Check sheet for the modelled part. Datum: model origin and axes. Units: mm. Give positions to 0.01 mm unless a question says otherwise; leave off trailing zeros. Order: outer loops, then holes, each group sorted by start corner. A loop starts at its lowest first (then second) coordinate and runs counter-clockwise, first axis right, second up. Notation, with made-up numbers: M 78.25,29 L 106.25,29 A7 ccw 106.25,36 Z; hole C -25,6.5 d2. An arc over 180 degrees is marked long. Return JSON: item names as keys, results as strings. Group by question number.
from build123d import *

# Parameters (mm, degrees)
BOSS_EXTRUDE1_DEPTH = 3
SKETCH2_W           = 249.6
SKETCH2_H           = 3
SKETCH2_W_2         = 14.577777778
SKETCH2_W_3         = 14.577777777
BOSS_EXTRUDE2_DEPTH = 3
BOSS_EXTRUDE5_DEPTH = 3
BOSS_EXTRUDE4_DEPTH = 3


with BuildPart() as part:
    # Sketch1 → Boss-Extrude1 (new body)
    with BuildSketch(Plane.XY):
        Polygon((-124.8, 111.588319146), (124.8, 111.588319146), (65, -111.588319146), (-65, -111.588319146), align=None)
    extrude(amount=BOSS_EXTRUDE1_DEPTH)

    # Sketch2 → Boss-Extrude2 (add, through all)
    with BuildSketch(Plane.XY.offset(3)):
        with Locations((0, 113.088319146)):
            Rectangle(SKETCH2_W, SKETCH2_H)
        with Locations((-57.711111111, -113.088319146)):
            Rectangle(SKETCH2_W_2, SKETCH2_H)
        with Locations((-28.855555556, -113.088319146)):
            Rectangle(SKETCH2_W_3, SKETCH2_H)
        with Locations((0, -113.088319146)):
            Rectangle(SKETCH2_W_2, SKETCH2_H)
        with Locations((28.855555556, -113.088319146)):
            Rectangle(SKETCH2_W_3, SKETCH2_H)
        with Locations((57.711111111, -113.088319146)):
            Rectangle(SKETCH2_W_2, SKETCH2_H)
    extrude(amount=-BOSS_EXTRUDE2_DEPTH)

    # Sketch4 → Boss-Extrude5 (add, through all)
    with BuildSketch(Plane.XY.offset(3)):
        Polygon((-124.8, 140.588319146), (-97.2, 140.588319146), (-97.2, 143.588319146), (-69.3, 143.588319146), (-69.3, 140.588319146), (-41.7, 140.588319146), (-41.7, 143.588319146), (-13.8, 143.588319146), (-13.8, 140.588319146), (13.8, 140.588319146), (13.8, 143.588319146), (41.7, 143.588319146), (41.7, 140.588319146), (69.3, 140.588319146), (69.3, 143.588319146), (97.2, 143.588319146), (97.2, 140.588319146), (124.8, 140.588319146), (127.8, 140.588319146), (127.8, 131.82165248), (124.8, 131.82165248), (124.8, 123.354985813), (127.8, 123.354985813), (127.8, 114.588319146), (124.8, 114.588319146), (-124.8, 114.588319146), (-127.8, 114.588319146), (-127.8, 123.354985813), (-124.8, 123.354985813), (-124.8, 131.82165248), (-127.8, 131.82165248), (-127.8, 140.588319146), align=None)
    extrude(amount=-BOSS_EXTRUDE5_DEPTH)

    # Sketch3 → Boss-Extrude4 (add, through all)
    with BuildSketch(Plane.XY.offset(3)):
        Polygon((127.8, 114.588319146), (124.8, 114.588319146), (124.8, 111.588319146), (118.12104635, 86.662124781), (120.920084455, 85.912124781), (127.8, 111.588319146), align=None)
        Polygon((74.477991756, -87.412124781), (71.67895365, -86.662124781), (65, -111.588319146), (65, -114.588319146), (67.196152423, -114.588319146), align=None)
        Polygon((87.758253344, -37.849513799), (84.959215238, -37.099513799), (78.280261587, -62.025708164), (81.079299693, -62.775708164), align=None)
        Polygon((101.038514931, 11.713097182), (98.239476825, 12.463097182), (91.560523175, -12.463097182), (94.35956128, -13.213097182), align=None)
        Polygon((114.318776518, 61.275708164), (111.519738413, 62.025708164), (104.840784762, 37.099513799), (107.639822868, 36.349513799), align=None)
        Polygon((-65, -111.588319146), (-71.67895365, -86.662124781), (-74.477991756, -87.412124781), (-67.196152423, -114.588319146), (-65, -114.588319146), align=None)
        Polygon((-78.280261587, -62.025708164), (-84.959215238, -37.099513799), (-87.758253344, -37.849513799), (-81.079299693, -62.775708164), align=None)
        Polygon((-91.560523175, -12.463097182), (-98.239476825, 12.463097182), (-101.038514931, 11.713097182), (-94.35956128, -13.213097182), align=None)
        Polygon((-104.840784762, 37.099513799), (-111.519738413, 62.025708164), (-114.318776518, 61.275708164), (-107.639822868, 36.349513799), align=None)
        Polygon((-127.8, 111.588319146), (-120.920084455, 85.912124781), (-118.12104635, 86.662124781), (-124.8, 111.588319146), (-124.8, 114.588319146), (-127.8, 114.588319146), align=None)
    extrude(amount=-BOSS_EXTRUDE4_DEPTH)


solid = part.part
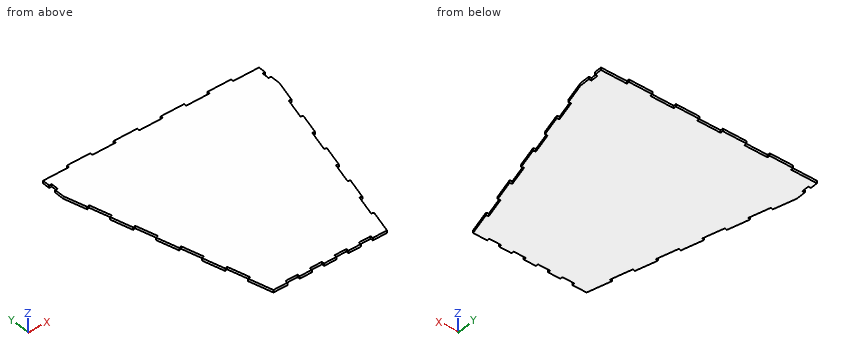
1) Material ranges on line 1 along Y through (x, z) = (-56.5, 0.4); line 2 along X through (y, z) = (-2.5, 0.6); line 3 along Y through (x, z) = (-20, 1.15), recorded low to high.
2) Depth check by flat-ended pin: P1, Ø0.9, axis at x = -49, z = 2, coming from the +Y side; P2, Ø1.5, axis at x = -12, z = 2, coming from the -Y side; P3, Ø0.9, axis at y = -114, z = 1, coming from the -X side. Enter the tip coordinate at first touch or a pass-through.
3) Sectioned sample at A-A on y = 44.5. Record the boundary of the cut face in (x, z), then the cut area to 3 significant figures.
4) Sectioned sample at B-B on y = -72. Record the boundary of the cut face in (x, z), then the cut area to 3 significant figures.
Reply:
{
 "1": {"line 1": "-114.59 to 140.59", "line 2": "-97.23 to 97.23", "line 3": "-111.59 to 143.59"},
 "2": {"P1": "y = 140.59", "P2": "y = -111.59", "P3": "x = -67.47"},
 "3": {"outline": "M -109.82,0 L 109.82,0 L 109.82,3 L -109.82,3 Z", "area": "659 mm^2"},
 "4": {"outline": "M -75.61,0 L 75.61,0 L 75.61,3 L -75.61,3 Z", "area": "454 mm^2"}
}
